Geometry: final body of the model. Coordinates: model frame, mm. A direction names the side the tool comes from. Give positions to 0.01 mm unless a question says otherwise; leave off trailing zeros. Loops run counter-clockwise (first coordinate to the right, second up) from the corner with the lowest first, then second, coordinate; pieces in that order, holes last.
1. Section A-A, the plane y = 45.5. Output: boundary loops of the cut face in (x, z), then the cut area to 3 significant figures.
2. Section C-C, the plane z = 8.5. Output: boundary loops of the cut face in (x, y).
3. Draft query along Y for faces 1 (the face through (0, 1, 0)), 2 (the face through (-2, 37.5, 8)), 3 (the face through (0, -67.5, 8)). Return one class per face: +Y half, -Y half, draft (parallel to the pull), parting line (faces both ways), or undercut.
4. Material intervals for line 1 along Y through (x, z) = (-8.5, 10.75); line 2 along X through (y, z) = (-5.5, 3.75); line 3 along X through (y, z) = (61.5, 1.5), sorted ascending.
5. Section B-B, the plane x = 2.5. Output: boundary loops of the cut face in (y, z), then the cut area to 3 significant figures.
6. Access query for faces 4 (the face through (-9, -15, 8)), 5 (the face through (-10, 1, 8)). Directions: +Z, -Z, +X, -X, +Y, -Y. A direction counts if a zero-diameter tool reaches every point of the face in a straight line with its end or side. Return the directions, or none.
7. Section D-D, the plane y = -25. Output: boundary loops of the cut face in (x, z), then the cut area to 3 significant figures.
from build123d import *

# Parameters (mm, degrees)
F0_W     = 20
F0_H     = 135
F1_DEPTH = 1
F2_W     = 18
F2_H     = 1
F3_DEPTH = 15


with BuildPart() as f1:
    # F0 (on Top) → F1 (new body)
    with BuildSketch(Plane.XY):
        Rectangle(F0_W, F0_H)
    extrude(amount=F1_DEPTH)

    # F2 (on face) → F3 (join)
    with BuildSketch(Plane.XY.offset(1)):
        Polygon((-10, -66.5), (-10, -67.5), (10, -67.5), (10, -66.5), (9, -66.5), (-9, -66.5), align=None)
        Polygon((-10, 67.5), (-10, -66.5), (-9, -66.5), (-9, 37.5), (-9, 38.5), (-9, 66.5), (-9, 67.5), align=None)
        Polygon((9, -66.5), (10, -66.5), (10, 67.5), (9, 67.5), (9, 66.5), align=None)
        with Locations((0, 67)):
            Rectangle(F2_W, F2_H)
        Polygon((-9, 38.5), (-9, 37.5), (6, 37.5), (6, -65.5), (7, -65.5), (7, 38.5), align=None)
    extrude(amount=F3_DEPTH)


solid = f1.part
Answers below:
1. outline: (-10, 0) - (10, 0) - (10, 16) - (9, 16) - (9, 1) - (-9, 1) - (-9, 16) - (-10, 16) - close
1. area: 50.0 mm2
2. outline: (-10, -67.5) - (10, -67.5) - (10, 67.5) - (-10, 67.5) - close; hole (-9, -66.5) - (9, -66.5) - (9, 66.5) - (-9, 66.5) - (-9, 38.5) - (7, 38.5) - (7, -65.5) - (6, -65.5) - (6, 37.5) - (-9, 37.5) - close
3. face 1: draft
3. face 2: undercut
3. face 3: -Y half
4. line 1: y = -67.5 to -66.5, 37.5 to 38.5, 66.5 to 67.5
4. line 2: x = -10 to -9, 6 to 7, 9 to 10
4. line 3: x = -10 to -9, 9 to 10
5. outline: (-67.5, 0) - (67.5, 0) - (67.5, 16) - (66.5, 16) - (66.5, 1) - (38.5, 1) - (38.5, 16) - (37.5, 16) - (37.5, 1) - (-66.5, 1) - (-66.5, 16) - (-67.5, 16) - close
5. area: 180 mm2
6. face 4: +Z
6. face 5: +Z, -Z, -X, +Y, -Y
7. outline: (-10, 0) - (10, 0) - (10, 16) - (9, 16) - (9, 1) - (7, 1) - (7, 16) - (6, 16) - (6, 1) - (-9, 1) - (-9, 16) - (-10, 16) - close
7. area: 65.0 mm2
